```python
from build123d import *

# Parameters (mm, degrees)
BOSS_EXTRUDE1_DEPTH = 38.1
SKETCH4_R           = 25.4
CUT_EXTRUDE1_DEPTH  = 684.562089353


with BuildPart() as part:
    # Sketch3 → Boss-Extrude1 (new, symmetric)
    with BuildSketch(Plane.XY):
        with BuildLine():
            Line((-228.6, -406.4), (-228.6, 330.2))
            Line((-228.6, 330.2), (25.03619311, 482.6))
            Line((25.03619311, 482.6), (254, 330.2))
            Line((254, 330.2), (254, -406.4))
            ThreePointArc((254, -406.4), (231.681536726, -460.281536726), (177.8, -482.6))
            Line((177.8, -482.6), (-152.4, -482.6))
            ThreePointArc((-152.4, -482.6), (-206.281536726, -460.281536726), (-228.6, -406.4))
        make_face()
    extrude(amount=BOSS_EXTRUDE1_DEPTH, both=True)

    # Sketch4 → Cut-Extrude1 (cut, through all)
    with BuildSketch(Plane.ZY.offset(228.6)):
        with Locations((0, 215.9)):
            Circle(SKETCH4_R)
        with Locations((0, -292.1)):
            Circle(SKETCH4_R)
    extrude(amount=-CUT_EXTRUDE1_DEPTH, mode=Mode.SUBTRACT)


solid = part.part
```
Model file for the job. Use its own axes, mm. Coordinates: 2 decimals unless noted, no trailing zeros. Loops run counter-clockwise (first coordinate to the right, second up) from the corner with the lowest first, then second, coordinate; pieces in that order, holes last. Notation, with made-up numbers: (39, 35.5) - (49, 35.5) arc R34 ccw to (49, 66.5) - close; hole circle Ø1 at (13.25, 82.25). An arc over 180 degrees is marked (long way). Answer as a JSON object with one key per item and string values. Group by question number.
(1) Cut at D-D (x = -137). Give the cut face in (y, z), then the cut area to 3 significant figures.
(2) Flat gauge pins, fed straight in: pin 1 (3 mm diameter, centred on x = 165, z = -26, fed in from +Y); pin 2 (3 mm diameter, centred on x = 65.5, z = 27, fed in from +Y). Where does each tip first touch, or does it go through?
(3) Cut at C-C (x = 58). Give the cut face in (y, z), then the cut area to 3 significant figures.
(4) Cut at A-A (z = 0). Give the cut face in (x, y), then the cut area to 3 significant figures.
(5) Cut at B-B (y = 215.9). Give the cut face in (x, z).
(6) Probe line 1 along Y through (x, z) = (-103, 0); line 2 along Y through (x, z) = (-84, 0); line 3 along Z through (x, y) = (-84, 215). List the from-to ranges inside material, lowest first.
(7) Two-plate mould, pull along Y, no slides. Class faces 1 (the face through (-205.686, -460.871, 0.533)), 2 (the face through (9.322, 193.366, 11.721)), 3 (the face through (-228.6, -43, 1)): released by +Y, released by -Y, zero draft, split by the parting line, or undercut.
Geometry says:
{
 "1": {"outline": "(-482.6, -38.1) - (385.24, -38.1) - (385.24, 38.1) - (-482.6, 38.1) - close; hole circle Ø50.8 at (-292.1, 0); hole circle Ø50.8 at (215.9, 0)", "area": "62,100 mm^2"},
 "2": {"pin 1": "stops at y = 390.44", "pin 2": "stops at y = 456.67"},
 "3": {"outline": "(-482.6, -38.1) - (460.66, -38.1) - (460.66, 38.1) - (-482.6, 38.1) - close; hole circle Ø50.8 at (-292.1, 0); hole circle Ø50.8 at (215.9, 0)", "area": "67,800 mm^2"},
 "4": {"outline": "(-228.6, -406.4) arc R76.2 ccw to (-152.4, -482.6) - (177.8, -482.6) arc R76.2 ccw to (254, -406.4) - (254, -317.5) - (-228.6, -317.5) - close; (-228.6, -266.7) - (254, -266.7) - (254, 190.5) - (-228.6, 190.5) - close; (-228.6, 241.3) - (254, 241.3) - (254, 330.2) - (25.04, 482.6) - (-228.6, 330.2) - close", "area": "378,000 mm^2"},
 "5": {"outline": "(-228.6, -38.1) - (254, -38.1) - (254, -25.4) - (-228.6, -25.4) - close; (-228.6, 25.4) - (254, 25.4) - (254, 38.1) - (-228.6, 38.1) - close"},
 "6": {"line 1": "y = -482.6 to -317.5, -266.7 to 190.5, 241.3 to 405.67", "line 2": "y = -482.6 to -317.5, -266.7 to 190.5, 241.3 to 417.08", "line 3": "z = -38.1 to -25.38, 25.38 to 38.1"},
 "7": {"face 1": "released by -Y", "face 2": "undercut", "face 3": "zero draft"}
}
